```python
from build123d import *

# Parameters (mm, degrees)
PAD_DEPTH       = 10
SKETCH001_R     = 1.5
POCKET_DEPTH    = 18.501
POCKET001_DEPTH = 2.4
SKETCH003_R     = 1.5
POCKET002_DEPTH = 38.001
POCKET003_DEPTH = 35


with BuildPart() as part:
    # Sketch → Pad (new body)
    with BuildSketch(Plane.XY):
        Polygon((0, 0), (30, 0), (30, 1.5), (38, 1.5), (38, 5.5), (30, 5.5), (4, 20), (0, 20), align=None)
    extrude(amount=PAD_DEPTH)

    # Sketch001 (on Face3 of Pad) → Pocket (cut, through all)
    with BuildSketch(Plane(origin=(30, 1.5, 0), x_dir=(1, 0, 0), z_dir=(0, -1, 0))):
        with Locations((4, 5)):
            Circle(SKETCH001_R)
    extrude(amount=-POCKET_DEPTH, mode=Mode.SUBTRACT)

    # Sketch002 (on Face9 of Pocket) → Pocket001 (cut)
    with BuildSketch(Plane(origin=(0, 5.5, 0), x_dir=(-1, 0, 0), z_dir=(0, 1, 0))):
        Polygon((-30.824574, 5), (-32.412287, 7.75), (-35.587713, 7.75), (-37.175426, 5), (-35.587713, 2.25), (-32.412287, 2.25), align=None)
    extrude(amount=-POCKET001_DEPTH, mode=Mode.SUBTRACT)

    # Sketch003 (on Face2 of Pocket001) → Pocket002 (cut, through all)
    with BuildSketch(Plane(origin=(0, 0, 0), x_dir=(0, -1, 0), z_dir=(-1, 0, 0))):
        with Locations((-15, 5)):
            Circle(SKETCH003_R)
    extrude(amount=-POCKET002_DEPTH, mode=Mode.SUBTRACT)

    # Sketch004 (on Face9 of Pocket002) → Pocket003 (cut)
    with BuildSketch(Plane.YZ.offset(38)):
        Polygon((16.587713, 2.25), (18.175426, 5), (16.587713, 7.75), (13.412287, 7.75), (11.824574, 5), (13.412287, 2.25), align=None)
    extrude(amount=-POCKET003_DEPTH, mode=Mode.SUBTRACT)


solid = part.part
```
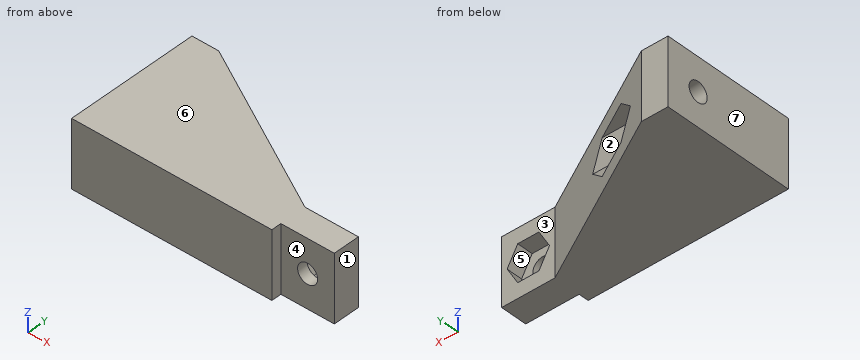
Verification items for the finished model (mm, model axes). Face numbers are marked on the shaded views. A direction names the side the tool comes from. Give positions to 0.01 mm unless a question says otherwise; leave off trailing zeros. Order: outer loops, then holes, each group sorted by start corner. A loop starts at its lowest first (then second) coordinate and runs counter-clockwise, first axis right, second up. Notation, with made-up numbers: (66.25, 57.5) -> (123.25, 57.5) arc R21 ccw to (123.25, 65.5) -> close; hole circle Ø2 at (23, -16). An arc over 180 degrees is marked (long way). Use a Markdown table: item, result.
1) Depth check by flat-ended pin: pin 1 Ø6 at (x, z) = (10, 8) entering from +Y; pin 2 Ø4 at (x, z) = (34, 5) entering from +Y; pin 3 Ø6 at (y, z) = (14, 6) entering from +X; pin 4 Ø2.5 at (x, z) = (34, 5) entering from +Y. Enter the tip coordinate at first touch or a pass-through.
Results:
| item | result |
|---|---|
| pin 1 | y = 18.33 |
| pin 2 | y = 3.1 |
| pin 3 | x = 20.14 |
| pin 4 | through |
2) Material ranges on probe 1 along Z at (x, y) = (0.65, 15); probe 2 along X at (y, z) = (14, 6.5); probe 3 along Y at (x, z) = (36, 2), recorded low to high.
Results:
| item | result |
|---|---|
| probe 1 | 0 to 3.5, 6.5 to 10 |
| probe 2 | 0 to 3 |
| probe 3 | 1.5 to 5.5 |
3) Tool access check on the marked faces 1, 2, 3 and 4. Record the directions out of +Z, -Z, +X, -X, +Y, -Y that give a thin tool (end or side, any length) a straight path to the whole face; none if there is none.
Results:
| item | result |
|---|---|
| face 1 | +Z, -Z, +X, +Y, -Y |
| face 2 | +X |
| face 3 | +Z, -Z, +X, +Y |
| face 4 | +Z, -Z, +X, -Y |
4) Section check C-C, the plane y = 12.5. Record the boundary of the cut face in (x, z), then the cut area to 3 significant figures.
Results:
| item | result |
|---|---|
| outline | (0, 0) -> (17.45, 0) -> (17.45, 3.83) -> (3, 3.83) -> (3, 6.17) -> (17.45, 6.17) -> (17.45, 10) -> (0, 10) -> close |
| area | 141 mm² |
5) Section check D-D, the plane x = 17. Record the boundary of the cut face in (y, z).
Results:
| item | result |
|---|---|
| outline | (0, 0) -> (12.75, 0) -> (12.75, 3.4) -> (11.82, 5) -> (12.75, 6.6) -> (12.75, 10) -> (0, 10) -> close |
6) Section check A-A, the plane x = 34. Record the boundary of the cut face in (y, z), then the cut area to 3 significant figures.
Results:
| item | result |
|---|---|
| outline | (1.5, 0) -> (5.5, 0) -> (5.5, 2.25) -> (3.1, 2.25) -> (3.1, 3.5) -> (1.5, 3.5) -> close; (1.5, 6.5) -> (3.1, 6.5) -> (3.1, 7.75) -> (5.5, 7.75) -> (5.5, 10) -> (1.5, 10) -> close |
| area | 22.0 mm² |
7) Section check B-B, the plane y = 14.5. Record the boundary of the cut face in (x, z).
Results:
| item | result |
|---|---|
| outline | (0, 0) -> (13.86, 0) -> (13.86, 2.25) -> (3, 2.25) -> (3, 3.59) -> (0, 3.59) -> close; (0, 6.41) -> (3, 6.41) -> (3, 7.75) -> (13.86, 7.75) -> (13.86, 10) -> (0, 10) -> close |
8) Mould release check, pull along Z, two halves, no side actions. Record for the marked faces 5, 6 and 7: pulls with the +Z half, pulls with the -Z half, needs draft (parallel to the pull), parting line crosses it, or undercut.
Results:
| item | result |
|---|---|
| face 5 | undercut |
| face 6 | pulls with the +Z half |
| face 7 | needs draft |
